Autodesk Inventor part; units mm, degrees
ref_plane "YZ Plane" through (0, 0, 0) normal (1, 0, 0) x (0, 1, 0)
ref_plane "XZ Plane" through (0, 0, 0) normal (0, 1, 0) x (-1, 0, 0)
ref_plane "XY Plane" through (0, 0, 0) normal (0, 0, 1) x (1, 0, 0)
sketch "Sketch1" plane through (0, 0, 0) normal (0, 0, 1) x (1, 0, 0)
  circle A0 centre (0, 0) radius 5.5
  circle A1 centre (0, 0) radius 3
  dimension "d0" = 11
  dimension "d1" = 6
extrude "tube" add sketch "Sketch1" along normal blind 530
sketch "Sketch2" plane through (0, 0, 0) normal (0, 1, 0) x (-1, 0, 0)
  line L0 (0, 0) -> (150, 0)
  line L1 (150, 0) -> (150, 530)
  line L2 (150, 530) -> (0, 530)
  line L3 (0, 530) -> (0, 0)
  line L4 (75, 0) -> (165.4178, 0) construction
  line L5 (74, 530) -> (150, 367.0175)
  line L6 (74, 530) -> (253.8313, 530) construction
  line L7 (150, 77.1972) -> (58, 0)
  point P0 (150, 333)
  dimension "d4" = 150
  dimension "d5" = 530
  dimension "d9" = 65
  dimension "d16" = 74
  dimension "d17" = 58
  dimension "d18" = 40
extrude "tail" add sketch "Sketch2" along normal mid plane 4 contours L3 L2 L5 L1 L7 L0
fillet "Fillet1" radius 40 4 edges at (-74, 0, 530) (-150, 0, 367.0175) (-150, 0, 77.1972) (-58, 0, 0)
fillet "Fillet2" radius 20 2 edges at (-5.1235, -2, 265) (-5.1235, 2, 265)
extrude "shaft" add sketch "Sketch1" along normal blind 560 and the other way blind 30 contours A1
equation "\"d2\" = tail_height"
equation "\"d5\" = tail_height"
properties part number "tail2"
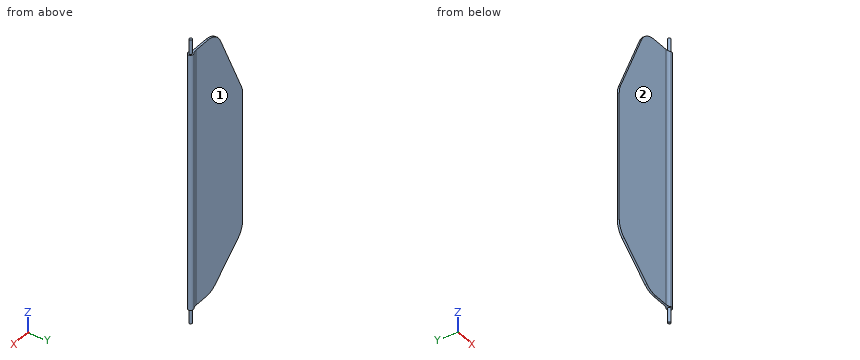
Geometry: final body of the model. Coordinates: model frame, mm. Face numbers are marked on the shaded views. A direction names the side the tool comes from. Give positions to 0.01 mm unless a question says otherwise; leave off trailing zeros. Write each loop counter-clockwise with the first axis right and the second up, starting at its lowest first coordinate (ties: lowest second). Pieces come first, ordered by that corner, then holes. Notation, with made-up numbers: (-2.5, 28) - (15.5, 28) arc R22 ccw to (15.5, 43) - close; hole circle Ø10 at (76, -17). An arc over 180 degrees is marked (long way). Return JSON: item names as keys, results as strings. Group by question number.
1) Section D-D on z = 401.5. Return the cut outline in (x, y), plus the area to 3 significant figures.
2) Section C-C on x = -33.5. Return the cut outline in (y, z), plus the area to 3 significant figures.
3) Section B-B on z = 289.5. Return the cut outline in (x, y), plus the area to 3 significant figures.
4) Set-up query: the marked faces 1 and 2. Return all of +Z, -Z, +X, -X, +Y, -Y with unobstructed straight access to the full face (end or side cutting, diameter ignored); none if empty.
5) First-contact query: P1, Ø1, axis at x = -44, y = 2, coming from the +Z side; P2, Ø6, axis at x = -96.5, y = -1.5, coming from the +Z side; P3, Ø5, axis at x = -62, y = -2.5, coming from the +Z side. Flat tips, straight axial feed; report the tip coordinate or a pass-through.
6) Section A-A on y = 0. Return the cut outline in (x, z).
7) Line query: line 1 (Y direction, x = -114, z = 199.5); line 2 (Z direction, x = -13, y = -1); line 3 (X direction, y = -0.5, z = 27.5). Output: solid intervals per line, ascending.
Filled in:
{
 "1": {"outline": "(-133.92, -2) - (-12.89, -2) arc R20 cw to (-2.78, -4.75) arc R5.5 ccw (long way) to (-2.78, 4.75) arc R20 cw to (-12.89, 2) - (-133.92, 2) - close", "area": "619 mm^2"},
 "2": {"outline": "(-2, 0) - (2, 0) - (2, 530) - (-2, 530) - close", "area": "2,120 mm^2"},
 "3": {"outline": "(-150, -2) - (-12.89, -2) arc R20 cw to (-2.78, -4.75) arc R5.5 ccw (long way) to (-2.78, 4.75) arc R20 cw to (-12.89, 2) - (-150, 2) - close", "area": "684 mm^2"},
 "4": {"face 1": "+Z, -Z, -X, +Y", "face 2": "+Z, -Z, -X, -Y"},
 "5": {"P1": "stops at z = 530", "P2": "stops at z = 488.18", "P3": "stops at z = 528.45"},
 "6": {"outline": "(-150, 95.85) arc R40 ccw to (-135.71, 65.21) - (-69.15, 9.36) arc R40 ccw to (-43.44, 0) - (-3, 0) - (-3, -30) - (3, -30) - (3, 0) - (5.5, 0) - (5.5, 530) - (3, 530) - (3, 560) - (-3, 560) - (-3, 530) - (-48.52, 530) arc R40 ccw to (-84.77, 506.9) - (-146.25, 375.05) arc R40 ccw to (-150, 358.15) - close"},
 "7": {"line 1": "y = -2 to 2", "line 2": "z = 0 to 530", "line 3": "x = -90.77 to 5.48"}
}
